Autodesk Inventor part; units mm, degrees
ref_plane "YZ Plane" through (0, 0, 0) normal (1, 0, 0) x (0, 1, 0)
ref_plane "XZ Plane" through (0, 0, 0) normal (0, 1, 0) x (-1, 0, 0)
ref_plane "XY Plane" through (0, 0, 0) normal (0, 0, 1) x (1, 0, 0)
sketch "Sketch1" plane through (0, 0, 0) normal (0, 0, 1) x (1, 0, 0)
  circle A0 centre (0, 0) radius 21
  circle A1 centre (0, 0) radius 15
  dimension "d0" = 42
  dimension "d1" = 30
extrude "Extrusion1" add sketch "Sketch1" along normal blind 7
sketch "Sketch2" plane through (0, 0, 7) normal (0, 0, 1) x (1, 0, 0)
  circle A0 centre (0, 0) radius 21
  circle A1 centre (0, 0) radius 15
  circle A2 centre (0, 0) radius 20
  circle A3 centre (0, 0) radius 16
  dimension "d4" = 1
  dimension "d5" = 1
extrude "Extrusion2" cut sketch "Sketch2" against normal blind 0.5 contours A2
sketch "Sketch3" plane through (0, 0, 0) normal (0, 0, -1) x (-1, 0, 0)
  circle A0 centre (0, 0) radius 20
  circle A1 centre (0, 0) radius 16
extrude "Extrusion3" cut sketch "Sketch3" against normal blind 0.5
properties part number "bearing_42x30x7"
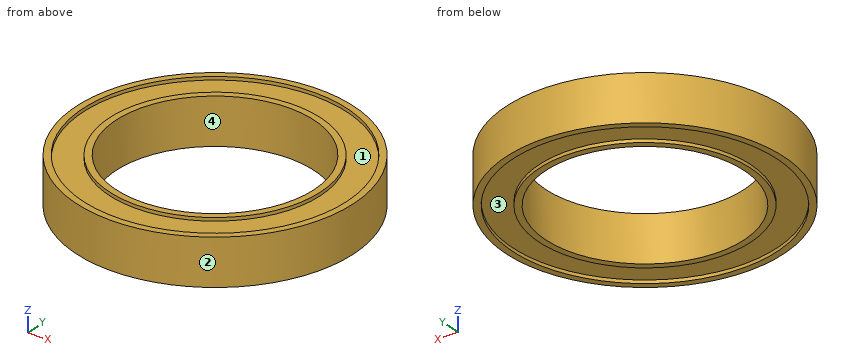
Here's how the part is built. I have some questions about the finished solid (model axes, mm). Face numbers are marked on the shaded views. A direction names the side the tool comes from. Coordinates: 2 decimals unless noted, no trailing zeros. Loops run counter-clockwise (first coordinate to the right, second up) from the corner with the lowest first, then second, coordinate; pieces in that order, holes last. Notation, with made-up numbers: (71.25, -3.75) -> (97.25, -3.75) arc R11 cw to (97.25, 13.25) -> close; hole circle Ø10 at (43, 36.25). An arc over 180 degrees is marked (long way). Use one line per item in the form item = value. Start each with the question number.
(1) Please list where these lines run through material, in increasing order: line 1 along Y through (x, z) = (0, 0.3); line 2 along Y through (x, z) = (0, 4.5); line 3 along X through (y, z) = (8, 6.25).
(2) If we section it at A-A (y = 0): Please give me the cut outline in (x, z), then the cut area to 3 significant figures.
(3) On a 3-axis mill with a long thin cutter (end or side, diameter ignored), from which of +Z, -Z, +X, -X, +Y, -Y can I reach the whole of each face in a straight line? I mean the marked faces 3 and 4. Say none if no direction works.
(4) If we section it at C-C (z = 2.5): Please give me the cut outline in (x, y).
(5) We'd pull the mould along X, two halves only. Please class the marked faces 1 and 2: pulls with the +X half, pulls with the -X half, needs draft (parallel to the pull), parting line crosses it, or undercut.
(6) If we section it at D-D (y = 17.5): Please give me the cut outline in (x, z), then the cut area to 3 significant figures.
(7) Will these pins go through, and if not, where does the flat tip stop? pin 1 (1.5 mm diameter, centred on y = -16, z = 3, fed in from -X); pin 2 (1 mm diameter, centred on x = -13, z = 4.5, fed in from -Y); pin 3 (20 mm diameter, centred on x = 7.5, y = -3.5, fed in from +Z); pin 4 (2 mm diameter, centred on y = 13, z = 2, fed in from +X).
Verdict:
q1.line_1 = -21 to -20, -16 to -15, 15 to 16, 20 to 21
q1.line_2 = -21 to -15, 15 to 21
q1.line_3 = -19.42 to -12.69, 12.69 to 19.42
q2.outline = (-21, 0) -> (-20, 0) -> (-20, 0.5) -> (-16, 0.5) -> (-16, 0) -> (-15, 0) -> (-15, 7) -> (-16, 7) -> (-16, 6.5) -> (-20, 6.5) -> (-20, 7) -> (-21, 7) -> close; (15, 0) -> (16, 0) -> (16, 0.5) -> (20, 0.5) -> (20, 0) -> (21, 0) -> (21, 7) -> (20, 7) -> (20, 6.5) -> (16, 6.5) -> (16, 7) -> (15, 7) -> close
q2.area = 76.0 mm²
q3.face_3 = -Z
q3.face_4 = +Z, -Z
q4.outline = circle Ø42 at (0, 0); hole circle Ø30 at (0, 0)
q5.face_1 = undercut
q5.face_2 = parting line crosses it
q6.outline = (-11.61, 0) -> (-9.68, 0) -> (-9.68, 0.5) -> (9.68, 0.5) -> (9.68, 0) -> (11.61, 0) -> (11.61, 7) -> (9.68, 7) -> (9.68, 6.5) -> (-9.68, 6.5) -> (-9.68, 7) -> (-11.61, 7) -> close
q6.area = 143 mm²
q7.pin_1 = -14.44
q7.pin_2 = -16.87
q7.pin_3 = 7
q7.pin_4 = 17.23
